Read the model definition and answer for the solid it produces. Units are mm, in the model's axes. A direction names the side the tool comes from. Coordinates: 2 decimals unless noted, no trailing zeros. Order: outer loops, then holes, each group sorted by start corner. A loop starts at its lowest first (then second) coordinate and runs counter-clockwise, first axis right, second up. Notation, with made-up numbers: (0.5, 32) - (43.5, 32) arc R29 ccw to (43.5, 70) - close; hole circle Ø2 at (-2, 46). An arc over 180 degrees is marked (long way). Write item = value, one per line.
from build123d import *

# Parameters (mm, degrees)
SKETCH1_R           = 2.5
SKETCH1_R_2         = 2.25
BOSS_EXTRUDE1_DEPTH = 16
SKETCH_2_W          = 51.4
SKETCH_2_H          = 4
EXTRUDE_1_DEPTH     = 55
SKETCH_3_R          = 2.25
CUT_EXTRUDE_2_DEPTH = 55
CUT_EXTRUDE_3_DEPTH = 11
CUT_EXTRUDE_START   = -27
CUT_EXTRUDE_4_DEPTH = 27
FILLET_1_R          = 4


with BuildPart() as part:
    # Sketch1 → Boss-Extrude1 (new, symmetric)
    with BuildSketch(Plane.XY):
        with BuildLine():
            Line((-21.2, 33), (-21.2, 22))
            Line((-21.2, 22), (-21.2, 0))
            Line((-21.2, 0), (-21.2, -4))
            Line((-21.2, -4), (30.2, -4))
            Line((30.2, -4), (30.2, 9))
            ThreePointArc((30.2, 9), (27.563961031, 15.363961031), (21.2, 18))
            Line((21.2, 18), (4.8, 18))
            ThreePointArc((4.8, 18), (-2.271067812, 20.928932188), (-5.2, 28))
            Line((-5.2, 28), (-5.2, 33))
            ThreePointArc((-5.2, 33), (-13.2, 41), (-21.2, 33))
        make_face()
        with Locations((21.2, 9)):
            Circle(SKETCH1_R, mode=Mode.SUBTRACT)
        with Locations((-13.2, 33)):
            Circle(SKETCH1_R_2, mode=Mode.SUBTRACT)
    extrude(amount=BOSS_EXTRUDE1_DEPTH, both=True)

    # 草图2 → 凸台-拉伸1 (add)
    with BuildSketch(Plane.XY.offset(16)):
        with Locations((4.5, -2)):
            Rectangle(SKETCH_2_W, SKETCH_2_H)
    extrude_1 = extrude(amount=EXTRUDE_1_DEPTH)

    # 草图3 → 切除-拉伸2 (cut)
    with BuildSketch(Plane(origin=(0, 0, 0), x_dir=(1, 0, 0), z_dir=(0, 1, 0))):
        with Locations(Location((11.5, -51, 0), (0, 0, 180))):
            Circle(SKETCH_3_R)
        with Locations(Location((4.5, -44, 0), (0, 0, 180))):
            Circle(SKETCH_3_R)
        with Locations(Location((4.5, -58, 0), (0, 0, 180))):
            Circle(SKETCH_3_R)
        with Locations(Location((-2.5, -51, 0), (0, 0, 180))):
            Circle(SKETCH_3_R)
        Polygon((30.2, -16), (20.2, -71), (30.2, -71), align=None)
        Polygon((-21.2, -16), (-11.2, -71), (-21.2, -71), align=None)
    cut_extrude_2 = extrude(amount=-CUT_EXTRUDE_2_DEPTH, mode=Mode.SUBTRACT)

    # 镜向1: 凸台-拉伸1, 切除-拉伸2 across plane
    add(extrude_1.mirror(Plane.XY))
    add(cut_extrude_2.mirror(Plane.XY), mode=Mode.SUBTRACT)

    # 草图6 → 切除-拉伸3 (cut, symmetric)
    with BuildSketch(Plane.XY):
        with BuildLine():
            Line((4.8, 18), (4.8, 0))
            Line((4.8, 0), (30.2, 0))
            Line((30.2, 0), (30.2, 9))
            ThreePointArc((30.2, 9), (27.563961031, 15.363961031), (21.2, 18))
            Line((21.2, 18), (4.8, 18))
        make_face()
    extrude(amount=CUT_EXTRUDE_3_DEPTH, both=True, mode=Mode.SUBTRACT)

    # 草图7 → 切除-拉伸4 (cut)
    with BuildSketch(Plane(origin=(0, 0, -16), x_dir=(-1, 0, 0), z_dir=(0, 0, -1)).offset(CUT_EXTRUDE_START)):
        with BuildLine():
            Line((-4.8, 18), (21.2, 18))
            Line((21.2, 18), (21.2, 33))
            ThreePointArc((21.2, 33), (13.2, 41), (5.2, 33))
            Line((5.2, 33), (5.2, 28))
            ThreePointArc((5.2, 28), (2.271067812, 20.928932188), (-4.8, 18))
        make_face()
    extrude(amount=CUT_EXTRUDE_4_DEPTH, mode=Mode.SUBTRACT)

    # 圆角1
    # the kernel refuses this fillet: 4 mm, written as the material it adds along each edge
    with BuildSketch(Plane(origin=(-31.2, 0, -16), x_dir=(0, 1, 0), z_dir=(1, 0, 0))) as fillet_1_piece_1_section:
        with BuildLine():
            CenterArc((FILLET_1_R, -FILLET_1_R), FILLET_1_R, 90, 90)
            Line((0, -FILLET_1_R), (0, 0))
            Line((0, 0), (FILLET_1_R, 0))
        make_face()
    fillet_1_piece_1 = extrude(amount=71.4, mode=Mode.PRIVATE)
    fillet_1_piece_1 = split(fillet_1_piece_1, bisect_by=Plane(origin=(-20.221053864, 0.89582788, -21.384203748), z_dir=(0.9838699100999075, 0, 0.178885438199983)), keep=Keep.TOP, mode=Mode.PRIVATE)
    fillet_1_piece_1 = split(fillet_1_piece_1, bisect_by=Plane(origin=(29.221053864, 0.89582788, -21.384203748), z_dir=(-0.9838699100999075, 0, 0.1788854381999831)), keep=Keep.TOP, mode=Mode.PRIVATE)
    add(fillet_1_piece_1)
    with BuildSketch(Plane(origin=(4.8, 18, 11), x_dir=(0, 1, 0), z_dir=(-1, 0, 0))) as fillet_1_piece_2_section:
        with BuildLine():
            CenterArc((FILLET_1_R, FILLET_1_R), FILLET_1_R, 180, 90)
            Line((0, FILLET_1_R), (0, 0))
            Line((0, 0), (FILLET_1_R, 0))
        make_face()
    fillet_1_piece_2 = extrude(amount=26, mode=Mode.PRIVATE)
    fillet_1_piece_2 = fillet_1_piece_2 - Plane(origin=(4.8, 28, 10.070813785), x_dir=(0, -1, 0), z_dir=(0, 0, 1)) * Cylinder(10, 68, mode=Mode.PRIVATE)
    add(fillet_1_piece_2)
    with BuildSketch(Plane(origin=(-31.2, 0, 16), x_dir=(0, 0, 1), z_dir=(1, 0, 0))) as fillet_1_piece_3_section:
        with BuildLine():
            CenterArc((FILLET_1_R, -FILLET_1_R), FILLET_1_R, 90, 90)
            Line((0, -FILLET_1_R), (0, 0))
            Line((0, 0), (FILLET_1_R, 0))
        make_face()
    fillet_1_piece_3 = extrude(amount=71.4, mode=Mode.PRIVATE)
    fillet_1_piece_3 = split(fillet_1_piece_3, bisect_by=Plane(origin=(29.221053864, 0.89582788, 21.384203748), z_dir=(-0.9838699100999075, 0, -0.1788854381999831)), keep=Keep.TOP, mode=Mode.PRIVATE)
    fillet_1_piece_3 = split(fillet_1_piece_3, bisect_by=Plane(origin=(-20.221053864, 0.89582788, 21.384203748), z_dir=(0.9838699100999075, 0, -0.178885438199983)), keep=Keep.TOP, mode=Mode.PRIVATE)
    add(fillet_1_piece_3)


solid = part.part
1) Determine the mould class of faces 5 (the face through (27.634, 15.294, 13.535)), 6 (the face through (4.79, -1.97, -46.23)), 7 (the face through (4.14, 1.141, 17.203)) for opening direction X: pulls with the +X half, pulls with the -X half, needs draft (parallel to the pull), parting line crosses it, or undercut.
Returned:
face_5 = pulls with the +X half
face_6 = undercut
face_7 = needs draft
2) Straight lines are drawn through the part: line 1 along Z through (x, y) = (11.5, -1.4); line 2 along Z through (x, y) = (9.5, 9.5); line 3 along X through (y, z) = (9, -13.4). For each, find the intervals that lie inside material, in ascending order. Write a range as from..to.
Returned:
line_1 = -71..-53.25, -48.75..48.75, 53.25..71
line_2 = -16..-11, 11..16
line_3 = -21.2..18.7, 23.7..30.2
3) Flat-ended cylindrical pins translate along their axes: pin 1 Ø5 at (x, z) = (11.5, 51) entering from +Y; pin 2 Ø3.5 at (x, z) = (4.5, 44) entering from +Y; pin 3 Ø6 at (x, y) = (21.2, 9) entering from -Z; pin 4 Ø14.5 at (x, y) = (-13, 32.5) entering from -Z. Find the tip coordinate at first contact, or state that the pin passes through.
Returned:
pin_1 = 0
pin_2 = through
pin_3 = -16
pin_4 = 11
4) For faces 1 (the face through (-2.21, -1.97, -53.23)), 2 (the face through (-2, 15, 16)), 3 (the face through (-5.2, 30, 14)), 4 (the face through (-4, 18, -7)), determine the directions among +Z, -Z, +X, -X, +Y, -Y from which every point of the face is accessible in a straight line to the end or side of a thin tool.
Returned:
face_1 = +Y, -Y
face_2 = +Z, +X, -X, +Y
face_3 = +Z, -Z, +X, +Y
face_4 = -Z, +X, -X, +Y
5) The part is cut by section A-A (x = 11.5). Determine the outline of the cut face in (y, z).
Returned:
outline = (-4, -71) - (0, -71) - (0, -53.25) - (-4, -53.25) - close; (-4, -48.75) - (0, -48.75) - (0, -20) arc R4 cw to (4, -16) - (18, -16) - (18, -11) - (0, -11) - (0, 11) - (18, 11) - (18, 16) - (4, 16) arc R4 cw to (0, 20) - (0, 48.75) - (-4, 48.75) - close; (-4, 53.25) - (0, 53.25) - (0, 71) - (-4, 71) - close
6) The part is cut by section C-C (z = -58). Determine the outline of the cut face in (x, y).
Returned:
outline = (-13.56, -4) - (2.25, -4) - (2.25, 0) - (-13.56, 0) - close; (6.75, -4) - (22.56, -4) - (22.56, 0) - (6.75, 0) - close
7) The part is cut by section D-D (x = 25.5). Determine the outline of the cut face in (y, z), and give its area (3 significant figures).
Returned:
outline = (-4, -41.85) - (0, -41.85) - (0, -20) arc R4 cw to (4, -16) - (16.91, -16) - (16.91, -11) - (0, -11) - (0, 11) - (16.91, 11) - (16.91, 16) - (4, 16) arc R4 cw to (0, 20) - (0, 41.85) - (-4, 41.85) - close
area = 511 mm^2
8) The part is cut by section B-B (z = -13). Determine the outline of the cut face in (x, y), and give its area (3 significant figures).
Returned:
outline = (-21.2, -4) - (30.2, -4) - (30.2, 9) arc R9 ccw to (21.2, 18) - (-21.2, 18) - close; hole circle Ø5 at (21.2, 9)
area = 1,090 mm^2
